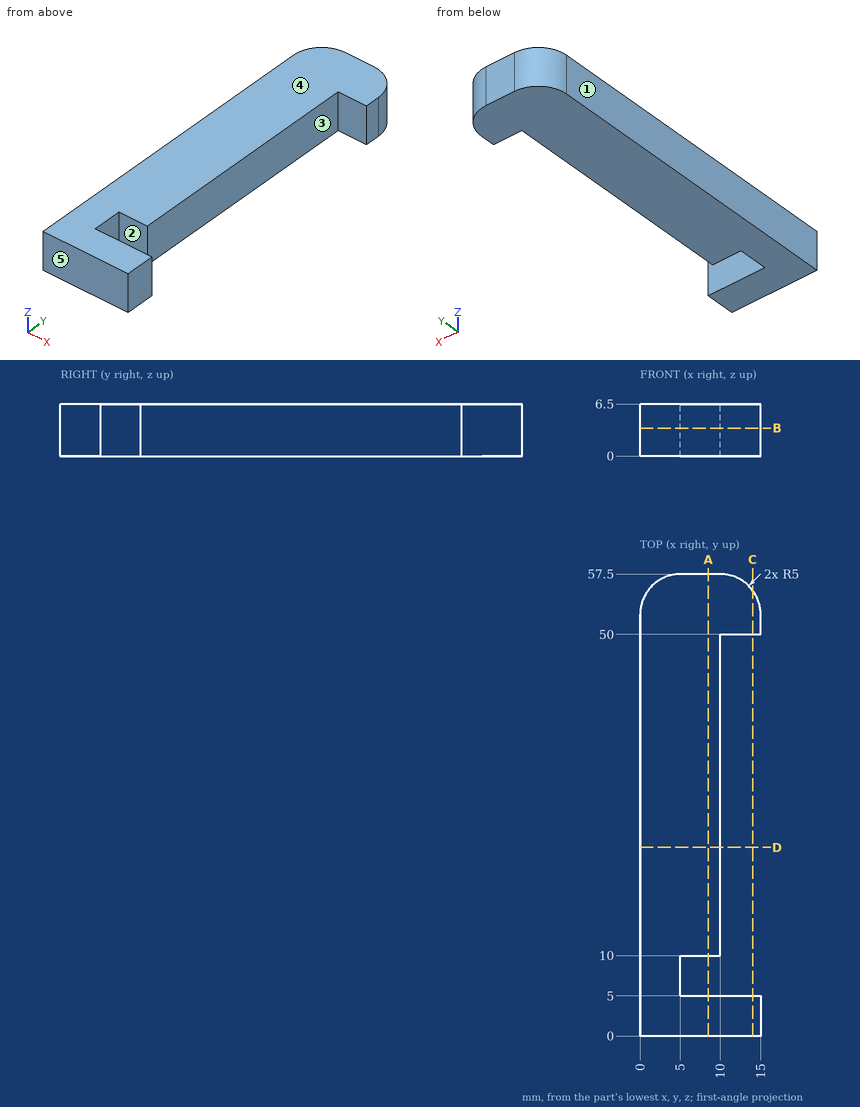
Design review of the part shown in the three views and the two pictorial views. Dimensions are in mm from the part's minimum x, y and z. A direction names the side the tool comes from. Round coordinates to 2 decimals unless told otherwise and drop trailing zeros. Loops run counter-clockwise (first coordinate to the right, second up) from the corner with the lowest first, then second, coordinate; pieces in that order, holes last.
1) Wall thickness on line 1 along Y through (x, z) = (8.75, 2.25); line 2 along Y through (x, z) = (10.25, 4); line 3 along X through (y, z) = (46, 2): over which ranges is each line inside the solid? List them lowest first.
Values follow:
line 1: y = 0 to 5, 10 to 57.5
line 2: y = 0 to 5, 50 to 57.49
line 3: x = 0 to 10
2) Tool access review of the marked faces 1 and 2: name each direction out of +Z, -Z, +X, -X, +Y, -Y from which nothing blocks a thin tool from reaching the whole face with its end or side.
Values follow:
face 1: +Z, -Z, -X, +Y, -Y
face 2: +Z, -Z, +X
3) Clearance check with flat-ended pins moving along their axes: P1, Ø3, axis at y = 20, z = 3, coming from the -X side; P2, Ø2, axis at y = 42.5, z = 5, coming from the +X side; P3, Ø1, axis at x = 12.5, y = 7, coming from the +Z side. State where each tip first meets the part, or that it passes through.
Values follow:
P1: stops at x = 0
P2: stops at x = 10
P3: passes through
4) Consider section A-A on x = 8.5. State the section outline as (y, z) points, then the cut area to 3 significant figures.
Values follow:
outline: (0, 0) - (5, 0) - (5, 6.5) - (0, 6.5) - close; (10, 0) - (57.5, 0) - (57.5, 6.5) - (10, 6.5) - close
area: 341 mm2
5) Consider section D-D on y = 23.5. State the section outline as (x, z) points, then the cut area to 3 significant figures.
Values follow:
outline: (0, 0) - (10, 0) - (10, 6.5) - (0, 6.5) - close
area: 65.0 mm2
6) The part is to be moulded in two halves that separate along Y. For the marked faces 3, 4 and 5, say which applies: pulls with the +Y half, pulls with the -Y half, needs draft (parallel to the pull), parting line crosses it, or undercut.
Values follow:
face 3: undercut
face 4: needs draft
face 5: pulls with the -Y half
7) Consider section B-B on z = 3.5. State the section outline as (x, y) points.
Values follow:
outline: (0, 0) - (15, 0) - (15, 5) - (5, 5) - (5, 10) - (10, 10) - (10, 50) - (15, 50) - (15, 52.5) arc R5 ccw to (10, 57.5) - (5, 57.5) arc R5 ccw to (0, 52.5) - close
8) Consider section C-C on x = 14. State the section outline as (y, z) points.
Values follow:
outline: (0, 0) - (5, 0) - (5, 6.5) - (0, 6.5) - close; (50, 0) - (55.5, 0) - (55.5, 6.5) - (50, 6.5) - close
